from build123d import *

# Parameters (mm, degrees)
SALIENTE_EXTRUIR6_DEPTH = 5.5
CROQUIS6_R              = 7
CORTAR_EXTRUIR1_DEPTH   = 11
CROQUIS10_OUTSIDE_W     = 69.118
CROQUIS10_OUTSIDE_H     = 65.714
CROQUIS10_OUTSIDE_R     = 10
CORTAR_EXTRUIR2_DEPTH   = 10
CORTAR_EXTRUIR2_DRAFT   = -60
CROQUIS11_OUTSIDE_W     = 69.118
CROQUIS11_OUTSIDE_H     = 65.714
CROQUIS11_OUTSIDE_R     = 10
CORTAR_EXTRUIR3_DEPTH   = 10
CORTAR_EXTRUIR3_DRAFT   = -60


with BuildPart() as part:
    # Croquis5 → Saliente-Extruir6 (new, symmetric)
    with BuildSketch(Plane(origin=(0, 0, 0), x_dir=(1, 0, 0), z_dir=(0, 1, 0))):
        Polygon((12.701705922, 0), (6.350852961, 11), (-6.350852961, 11), (-12.701705922, 0), (-6.350852961, -11), (6.350852961, -11), align=None)
    extrude(amount=SALIENTE_EXTRUIR6_DEPTH, both=True)

    # Croquis6 → Cortar-Extruir1 (cut)
    with BuildSketch(Plane(origin=(0, 5.5, 0), x_dir=(1, 0, 0), z_dir=(0, 1, 0))):
        with Locations(Location((0, 0, 0), (0, 0, 270))):
            Circle(CROQUIS6_R)
    extrude(amount=-CORTAR_EXTRUIR1_DEPTH, mode=Mode.SUBTRACT)


with BuildPart() as cortar_extruir2_tool:
    # Croquis10 outside → Cortar-Extruir2 (with draft: the straight prism first)
    with BuildSketch(Plane(origin=(0, 5.5, 0), x_dir=(1, 0, 0), z_dir=(0, 1, 0))):
        Rectangle(CROQUIS10_OUTSIDE_W, CROQUIS10_OUTSIDE_H)
        Circle(CROQUIS10_OUTSIDE_R, mode=Mode.SUBTRACT)
    extrude(amount=-CORTAR_EXTRUIR2_DEPTH)
    # Cortar-Extruir2: the draft: its side faces are tilted about the plane it starts from
    cortar_extruir2_sides = [cortar_extruir2_tool.faces().sort_by_distance(p)[0] for p in [
        (0, 0.5, 32.857),
        (34.559, 0.5, 0),
        (0, 0.5, -32.857),
        (-34.559, 0.5, 0),
        (-10, 0.5, 0),
    ]]
    draft(cortar_extruir2_sides, Plane(origin=(0, 5.5, 0), x_dir=(1, 0, 0), z_dir=(0, 1, 0)), CORTAR_EXTRUIR2_DRAFT)


with BuildPart() as part_1:
    add(part.part)

    # Cortar-Extruir2: cut by cortar_extruir2_tool
    add(cortar_extruir2_tool.part, mode=Mode.SUBTRACT)


with BuildPart() as cortar_extruir3_tool:
    # Croquis11 outside → Cortar-Extruir3 (with draft: the straight prism first)
    with BuildSketch(Plane.XZ.offset(5.5)):
        Rectangle(CROQUIS11_OUTSIDE_W, CROQUIS11_OUTSIDE_H)
        Circle(CROQUIS11_OUTSIDE_R, mode=Mode.SUBTRACT)
    extrude(amount=-CORTAR_EXTRUIR3_DEPTH)
    # Cortar-Extruir3: the draft: its side faces are tilted about the plane it starts from
    cortar_extruir3_sides = [cortar_extruir3_tool.faces().sort_by_distance(p)[0] for p in [
        (0, -0.5, -32.857),
        (34.559, -0.5, 0),
        (0, -0.5, 32.857),
        (-34.559, -0.5, 0),
        (-10, -0.5, 0),
    ]]
    draft(cortar_extruir3_sides, Plane.XZ.offset(5.5), CORTAR_EXTRUIR3_DRAFT)


with BuildPart() as part_2:
    add(part_1.part)

    # Cortar-Extruir3: cut by cortar_extruir3_tool
    add(cortar_extruir3_tool.part, mode=Mode.SUBTRACT)


solid = part_2.part
Could you check a few things on this model? Use its own coordinates, in mm. Round coordinates to 2 decimals unless told otherwise and drop trailing zeros. Loops run counter-clockwise (first coordinate to the right, second up) from the corner with the lowest first, then second, coordinate; pieces in that order, holes last. Notation, with made-up numbers: (-10, 53) - (5, 53) arc R4 cw to (5, 57) - close; hole circle Ø5 at (10, 82.25). An arc over 180 degrees is marked (long way). Write item = value, one per line.
1) Imagine slicing it at B-B (x = 0). Please give me the cut outline in (y, z).
Computed:
outline = (-5.5, -10) - (-4.92, -11) - (4.92, -11) - (5.5, -10) - (5.5, -7) - (-5.5, -7) - close; (-5.5, 7) - (5.5, 7) - (5.5, 10) - (4.92, 11) - (-4.92, 11) - (-5.5, 10) - close
2) If we mould it in two halves opening along X, with no side actions, what happens to faces 1 (the conical face through (9.663, 5.424, -3.043)), 2 (the flat face through (0, 0, 11)), 3 (the cylindrical face through (-6.834, 0.077, -1.517)), 4 (the flat face through (9.571, 0.069, -5.423))? For each: pulls with the +X half, pulls with the -X half, needs draft (parallel to the pull), parting line crosses it, or undercut.
Computed:
face_1 = parting line crosses it
face_2 = needs draft
face_3 = undercut
face_4 = pulls with the +X half
3) I need wall thicknesses on line 1 along Z through (x, y) = (-1.5, 1.5); line 2 along Z through (x, y) = (0.75, 2.75); line 3 along X through (y, z) = (1.5, 3.75). Which ranges of each line are inside material? Lowest first, please. Write a range as from..to.
Computed:
line_1 = -11..-6.84, 6.84..11
line_2 = -11..-6.96, 6.96..11
line_3 = -10.54..-5.91, 5.91..10.54
4) Imagine slicing it at A-A (y = -0.75). Please give me the cut outline in (x, z), and give its area (3 significant figures).
Computed:
outline = (-12.7, 0) - (-6.35, -11) - (6.35, -11) - (12.7, 0) - (6.35, 11) - (-6.35, 11) - close; hole circle Ø14 at (0, 0)
area = 265 mm2
5) I'm going to push flat-ended pins straight in: P1, Ø12.5, axis at x = 0, z = 0, coming from the +Y side; P2, Ø3, axis at x = -10, y = -3, coming from the -Z side; P3, Ø1, axis at y = 3, z = -3, coming from the +X side; P4, Ø2, axis at y = -2.5, z = -1.5, coming from the +X side. Where does each tip first touch, or does it pass through?
Computed:
P1 = through
P2 = -7.28
P3 = 11.26
P4 = 12.41
